```python
from build123d import *

# Parameters (mm, degrees)
BASEHEAD_DEPTH  = 2.925
SKETCH3_R       = 2
BASEBODY_DEPTH  = 8
CHAMFER1_SIZE   = 0.379
SKETCH5_W       = 1
SKETCH5_H       = 1.2
SLOT_DEPTH      = 4.39
SLOT_DEPTH_BACK = 4.39


with BuildPart() as part:
    # Sketch-BaseHead → BaseHead (new body)
    with BuildSketch(Plane(origin=(0, 0, 0), x_dir=(0, 0, -1), z_dir=(1, 0, 0))):
        Polygon((1.957217413, -3.39), (3.914434825, 0), (1.957217413, 3.39), (-1.957217413, 3.39), (-3.914434825, 0), (-1.957217413, -3.39), align=None)
    extrude(amount=BASEHEAD_DEPTH)

    # Sketch1 → Revolve1 (revolve)
    with BuildSketch(Plane.XY):
        Polygon((2.925, 0), (3.425, 0), (3.425, -2.94), (2.925, -3.39), align=None)
    revolve(axis=Axis((-4.001564945, 0, 0), (1, 0, 0)))

    # Sketch3 → BaseBody (add)
    with BuildSketch(Plane(origin=(3.425, 0, 0), x_dir=(0, 0, -1), z_dir=(1, 0, 0))):
        Circle(SKETCH3_R)
    extrude(amount=BASEBODY_DEPTH)

    # Chamfer1
    chamfer1_edges = [part.edges().sort_by_distance(p)[0] for p in [
        (11.425, 0, 2),
    ]]
    chamfer(chamfer1_edges, length=CHAMFER1_SIZE)

    # Sketch4 → HeadChamfer (revolve, cut)
    with BuildSketch(Plane(origin=(-0.264637255, 0, 5.916896391), x_dir=(0, 0, -1), z_dir=(0, 1, 0))):
        Polygon((9.831331216, -0.264637255), (9.306896391, -0.264637255), (9.831331216, -0.455515922), align=None)
    revolve(axis=Axis((-4.001564945, 0, 0), (1, 0, 0)), mode=Mode.SUBTRACT)

    # Sketch5 → Slot (cut, two sides)
    with BuildSketch(Plane(origin=(0, 0, 0), x_dir=(1, 0, 0), z_dir=(0, 1, 0))) as slot_sk:
        with Locations((0.5, 0)):
            Rectangle(SKETCH5_W, SKETCH5_H)
    extrude(amount=SLOT_DEPTH, mode=Mode.SUBTRACT)
    extrude(slot_sk.sketch, amount=-SLOT_DEPTH_BACK, mode=Mode.SUBTRACT)


solid = part.part
```
For this review, take the finished solid that the model builds, in its own axes (mm). A direction names the side the tool comes from. Round coordinates to 2 decimals unless told otherwise and drop trailing zeros. Order: outer loops, then holes, each group sorted by start corner. A loop starts at its lowest first (then second) coordinate and runs counter-clockwise, first axis right, second up.
Q1. Machinability: for faces 4 (the flat face through (2.925, -3, -2)), 5 (the flat face through (1, 0, 0)), 6 (the flat face through (2.925, -3, 2)), 7 (the flat face through (2.925, 3, -2)), 8 (the cylindrical face through (7, -2, 0)), which of the approach directions +Z, -Z, +X, -X, +Y, -Y give a long, thin tool a straight path to every point of the face, cutting with its end or side? Answer none if there is none.
Findings below:
face 4: -Z, +X, -Y
face 5: -X, +Y, -Y
face 6: +Z, +X, -Y
face 7: -Z, +X, +Y
face 8: +X
Q2. We need section B-B, the plane x = 9.5. Give the boundary of the cut face in (y, z).
Findings below:
outline: circle Ø4 at (0, 0)
Q3. We need section A-A, the plane x = 1.5. Give the boundary of the cut face in (y, z).
Findings below:
outline: (-3.39, -1.96) - (0, -3.91) - (3.39, -1.96) - (3.39, 1.96) - (0, 3.91) - (-3.39, 1.96) - close
Q4. Wall thickness on line 1 (X direction, y = 0, z = -0.25) (3 decimals); line 2 (Z direction, x = 8.5, y = 1); line 3 (Z direction, x = 3.75, y = -1.25): over which ranges is each line inside the solid? List them lowest first.
Findings below:
line 1: x = 1 to 11.425
line 2: z = -1.73 to 1.73
line 3: z = -1.56 to 1.56
Q5. Insertion check: P1, Ø1.4, axis at y = 3, z = 1.5, coming from the +X side (3 decimals); P2, Ø2, axis at x = 4, z = -0.5, coming from the -Y side; P3, Ø2, axis at x = 1, y = -2.5, coming from the +Z side. Each pin has a flat end and moves straight along its axis. Give the tip position at first contact, or say it passes through.
Findings below:
P1: stops at x = 3.425
P2: stops at y = -3.29
P3: stops at z = 3.05
Q6. Mouldability with a two-part tool opening along Z and no side actions: class faces 1 (the flat face through (0, 0, -2)), 2 (the flat face through (0.5, 0, -0.6)), 3 (the conical face through (0.054, 3.092, 1.722)) as pulls with the +Z half, pulls with the -Z half, needs draft (parallel to the pull), parting line crosses it, or undercut.
Findings below:
face 1: needs draft
face 2: undercut
face 3: pulls with the +Z half
